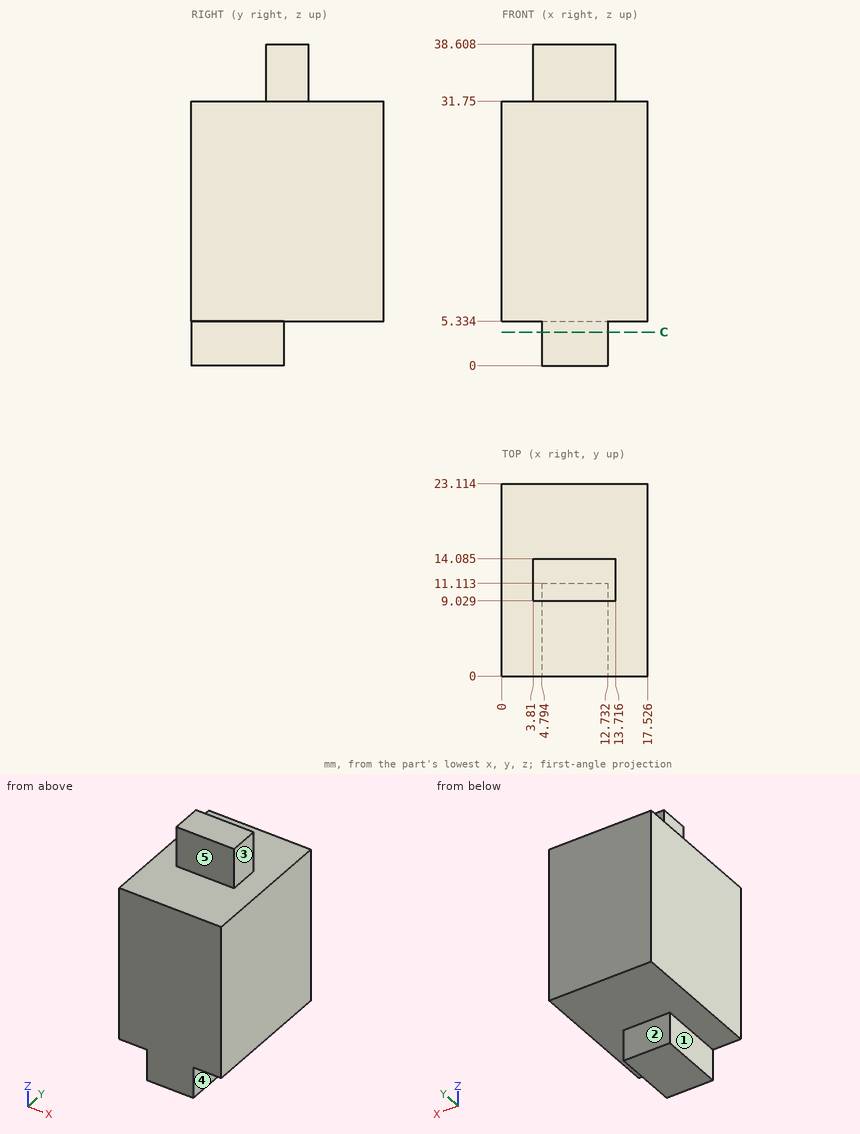
Geometry: see drawing. Coordinates: mm, zero at the bounding-box minimum. A direction names the side the tool comes from. Give positions to 0.01 mm unless a question says otherwise; leave off trailing zeros. Loops run counter-clockwise (first coordinate to the right, second up) from the corner with the lowest first, then second, coordinate; pieces in that order, holes last. Notation, with made-up numbers: (3.5, -34) -> (30.5, -34) arc R25 cw to (30.5, -6) -> close; hole circle Ø9 at (-15, 47). An arc over 180 degrees is marked (long way). Use one line per item in the form item = value.
Item 1: Pin query (flat end, axial travel): P1, Ø4.5, axis at x = 8, z = 2.5, coming from the +Y side; P2, Ø8, axis at y = 5.5, z = 4.5, coming from the -X side; P3, Ø4, axis at x = 14.5, y = 17.5, coming from the +Z side; P4, Ø2.5, axis at y = 12, z = 35, coming from the -X side. Return the tip coordinate at first contact, or that it passes through.
A:
P1 = 11.11
P2 = 0
P3 = 31.75
P4 = 3.81
Item 2: Section query C-C on z = 4. Output: boundary loops of the cut face in (x, y) (1 decimal).
A:
outline = (4.8, 0) -> (12.7, 0) -> (12.7, 11.1) -> (4.8, 11.1) -> close
Item 3: Access query for the marked faces 1, 2, 3, 4 and 5. Directions: +Z, -Z, +X, -X, +Y, -Y. A direction counts if a zero-diameter tool reaches every point of the face in a straight line with its end or side. Return the directions, or none.
A:
face_1 = -Z, -X, +Y, -Y
face_2 = -Z, +X, -X, +Y
face_3 = +Z, +X, +Y, -Y
face_4 = -Z, +X, +Y, -Y
face_5 = +Z, +X, -X, -Y
Item 4: Line query: probe 1 along Y at (x, z) = (11.5, 33.5) (1 decimal); probe 2 along Z at (x, y) = (5.5, 6.25); probe 3 along Z at (x, y) = (8, 13) (1 decimal). Output: solid intervals per line, ascending.
A:
probe_1 = 9 to 14.1
probe_2 = 0 to 31.75
probe_3 = 5.3 to 38.6
